CAD build for the part. Positions are in the model's coordinates, mm. A direction names the side the tool comes from. Round coordinates to 2 decimals unless told otherwise and drop trailing zeros. Write each loop counter-clockwise with the first axis right and the second up, starting at its lowest first coordinate (ties: lowest second). Pieces come first, ordered by that corner, then holes. Notation, with made-up numbers: (3, -9) - (27, -9) arc R17 cw to (27, 17) - close; hole circle Ø2 at (26.25, -8.75). An arc over 180 degrees is marked (long way). Answer in a Markdown table with one row per item.
```python
from build123d import *

# Parameters (mm, degrees)
ESQUISSE1_W                                        = 11
ESQUISSE1_H                                        = 26
BOSS_EXTRU_1_DEPTH                                 = 9
CHAMBRAGE_POUR_VIS_T_TE_RONDE_BOMB_E_M_D           = 3.4
CHAMBRAGE_POUR_VIS_T_TE_RONDE_BOMB_E_M_CBORE_D     = 7
CHAMBRAGE_POUR_VIS_T_TE_RONDE_BOMB_E_M_CBORE_DEPTH = 2.4
BOSS_EXTRU_2_DEPTH                                 = 40
DIAM_TRE_DU_PER_AGE_4_5_4_5_1_D                    = 4.5
ESQUISSE20_W                                       = 11
ESQUISSE20_H                                       = 28
ENL_V_MAT_EXTRU_6_DEPTH                            = 78.776924598
ESQUISSE21_W                                       = 50
ESQUISSE21_H                                       = 34
ENL_V_MAT_EXTRU_7_DEPTH                            = 72.960058366
ESQUISSE23_W                                       = 11
ESQUISSE23_H                                       = 14
BOSS_EXTRU_3_DEPTH                                 = 37
ESQUISSE24_W                                       = 37
ESQUISSE24_H                                       = 40
BOSS_EXTRU_4_DEPTH                                 = 3
ESQUISSE27_W                                       = 11
ESQUISSE27_H                                       = 37
ENL_V_MAT_EXTRU_11_DEPTH                           = 8
ESQUISSE28_W                                       = 64
ESQUISSE28_H                                       = 15
ENL_V_MAT_EXTRU_12_DEPTH                           = 6
ESQUISSE30_W                                       = 15
ESQUISSE30_H                                       = 8
ENL_V_MAT_EXTRU_13_DEPTH                           = 77.282370178
BOSS_EXTRU_6_DEPTH                                 = 3


with BuildPart() as part:
    # Esquisse1 → Boss.-Extru.1 (new body)
    with BuildSketch(Plane.XY):
        Rectangle(ESQUISSE1_W, ESQUISSE1_H)
    extrude(amount=BOSS_EXTRU_1_DEPTH)

    # Chambrage pour vis _ t_te ronde bomb_e M (through all)
    with Locations(Plane.XY.offset(9)):
        with Locations((0, 7.5), (0, -7.5)):
            CounterBoreHole(CHAMBRAGE_POUR_VIS_T_TE_RONDE_BOMB_E_M_D / 2, CHAMBRAGE_POUR_VIS_T_TE_RONDE_BOMB_E_M_CBORE_D / 2, CHAMBRAGE_POUR_VIS_T_TE_RONDE_BOMB_E_M_CBORE_DEPTH)

    # Esquisse8 → Boss.-Extru.2 (add)
    with BuildSketch(Plane.XZ.offset(13)):
        Polygon((-55.5, 0), (-55.5, 37), (5.5, 37), (5.5, 9), (-5.5, 9), (-5.5, 0), align=None)
    extrude(amount=-BOSS_EXTRU_2_DEPTH)

    # Diam_tre du per_age _4.5 _4.5_1 (through all)
    with Locations(Plane(origin=(0, 27, 0), x_dir=(1, 0, 0), z_dir=(0, 1, 0))):
        with Locations((-41.801370091, -19.00055804), (-18.801370091, -29.00055804)):
            Hole(DIAM_TRE_DU_PER_AGE_4_5_4_5_1_D / 2)

    # Esquisse20 → Enl_v. mat.-Extru.6 (cut, through all)
    with BuildSketch(Plane(origin=(0, 27, 0), x_dir=(1, 0, 0), z_dir=(0, 1, 0))):
        with Locations((0, -23)):
            Rectangle(ESQUISSE20_W, ESQUISSE20_H)
    extrude(amount=-ENL_V_MAT_EXTRU_6_DEPTH, mode=Mode.SUBTRACT)

    # Esquisse21 → Enl_v. mat.-Extru.7 (cut, through all)
    with BuildSketch(Plane.XY.offset(37)):
        with Locations((-30.5, 4)):
            Rectangle(ESQUISSE21_W, ESQUISSE21_H)
    extrude(amount=-ENL_V_MAT_EXTRU_7_DEPTH, mode=Mode.SUBTRACT)


with BuildPart() as enl_v_mat_extru_7_piece_1:
    # of the separate pieces the step leaves, piece 1, a body of its own (enl_v_mat_extru_7_pieces)
    add(part.part.solids().sort_by_distance((-5.5, 21, 0))[0])



with BuildPart() as enl_v_mat_extru_7_piece_2:
    # of the separate pieces the step leaves, piece 2, a body of its own (enl_v_mat_extru_7_pieces)
    add(part.part.solids().sort_by_distance((5.5, 13, 0))[0])


with BuildPart() as enl_v_mat_extru_7_piece_1_1:
    add(enl_v_mat_extru_7_piece_1.part)

    add(enl_v_mat_extru_7_piece_2.part)  # Boss.-Extru.3 merges Enl_v. mat.-Extru.7 piece 2
    # Esquisse23 → Boss.-Extru.3 (add, through all)
    with BuildSketch(Plane.XY.offset(37)):
        with Locations((0, 20)):
            Rectangle(ESQUISSE23_W, ESQUISSE23_H)
    extrude(amount=-BOSS_EXTRU_3_DEPTH)

    # Esquisse24 → Boss.-Extru.4 (add)
    with BuildSketch(Plane(origin=(5.5, 0, 0), x_dir=(0, 0, -1), z_dir=(1, 0, 0))):
        with Locations((-18.5, 7)):
            Rectangle(ESQUISSE24_W, ESQUISSE24_H)
    extrude(amount=BOSS_EXTRU_4_DEPTH)

    # Esquisse27 → Enl_v. mat.-Extru.11 (cut)
    with BuildSketch(Plane.XZ.offset(-21)):
        with Locations((0, 18.5)):
            Rectangle(ESQUISSE27_W, ESQUISSE27_H)
    extrude(amount=ENL_V_MAT_EXTRU_11_DEPTH, mode=Mode.SUBTRACT)

    # Esquisse28 → Enl_v. mat.-Extru.12 (cut)
    with BuildSketch(Plane(origin=(0, 27, 0), x_dir=(1, 0, 0), z_dir=(0, 1, 0))):
        with Locations((-23.5, -7.5)):
            Rectangle(ESQUISSE28_W, ESQUISSE28_H)
    extrude(amount=-ENL_V_MAT_EXTRU_12_DEPTH, mode=Mode.SUBTRACT)

    # Esquisse30 → Enl_v. mat.-Extru.13 (cut, through all)
    with BuildSketch(Plane.ZY.offset(-5.5)):
        with Locations((7.5, 17)):
            Rectangle(ESQUISSE30_W, ESQUISSE30_H)
    extrude(amount=-ENL_V_MAT_EXTRU_13_DEPTH, mode=Mode.SUBTRACT)

    # Esquisse31 → Boss.-Extru.6 (add, through all)
    with BuildSketch(Plane.ZY.offset(-5.5)):
        Polygon((15, 27), (0, 13), (15, 13), align=None)
    extrude(amount=-BOSS_EXTRU_6_DEPTH)


solid = enl_v_mat_extru_7_piece_1_1.part
```
Q1. Drill centre lines: line 1 (Y direction, x = 0, z = 7.25); line 2 (Y direction, x = 0, z = 2); line 3 (X direction, y = -10.5, z = 27.5). Where is each one in solid material? Low to high.
Computed:
| item | result |
|---|---|
| line 1 | y = -13 to -11, -4 to 4, 11 to 13 |
| line 2 | y = -13 to -9.2, -5.8 to 5.8, 9.2 to 13 |
| line 3 | x = 5.5 to 8.5 |
Q2. Saw through at D-D on y = 24. List the corners of the cut face in (x, z).
Computed:
| item | result |
|---|---|
| outline | (-55.5, 15) - (5.5, 15) - (5.5, 11.79) - (8.5, 11.79) - (8.5, 37) - (-55.5, 37) - close; hole circle Ø4.5 at (-41.8, 19); hole circle Ø4.5 at (-18.8, 29) |
Q3. 3-axis set-ups, long thin cutter, end or side, ignore diameter. For faces 1 (the flat face through (0, 13, 4)), 2 (the flat face through (-25, 21, 26)), 3 (the flat face through (2, 8, 6.6)): which of +Z, -Z, +X, -X, +Y, -Y reach the whole face in a straight line?
Computed:
| item | result |
|---|---|
| face 1 | +Z, -Z, -X, +Y |
| face 2 | +Z, -Z, -X, -Y |
| face 3 | +Z |
Q4. Saw through at B-B on y = -7.5. List the corners of the cut face in (x, z), then the cut area to 3 significant figures.
Computed:
| item | result |
|---|---|
| outline | (-5.5, 0) - (-1.7, 0) - (-1.7, 6.6) - (-3.5, 6.6) - (-3.5, 9) - (-5.5, 9) - close; (1.7, 0) - (8.5, 0) - (8.5, 37) - (5.5, 37) - (5.5, 9) - (3.5, 9) - (3.5, 6.6) - (1.7, 6.6) - close |
| area | 171 mm2 |
Q5. Saw through at C-C on z = 25.5. List the corners of the cut face in (x, y).
Computed:
| item | result |
|---|---|
| outline | (-55.5, 21) - (5.5, 21) - (5.5, -13) - (8.5, -13) - (8.5, 27) - (-55.5, 27) - close |
Q6. Flat gauge pins, fed straight in: pin 1 (2 mm diameter, centred on x = 1.5, y = -7.5, fed in from +Z); pin 2 (8 mm diameter, centred on y = 3, z = 28, fed in from -X); pin 3 (10 mm diameter, centred on x = -31.5, z = 26, fed in from -Y). Where does each tip first touch, or does it go through?
Computed:
| item | result |
|---|---|
| pin 1 | stops at z = 6.6 |
| pin 2 | stops at x = 5.5 |
| pin 3 | stops at y = 21 |
Q7. Saw through at A-A on x = 0. List the corners of the cut face in (y, z), then the cut area to 3 significant figures.
Computed:
| item | result |
|---|---|
| outline | (-13, 0) - (-9.2, 0) - (-9.2, 6.6) - (-11, 6.6) - (-11, 9) - (-13, 9) - close; (-5.8, 0) - (5.8, 0) - (5.8, 6.6) - (4, 6.6) - (4, 9) - (-4, 9) - (-4, 6.6) - (-5.8, 6.6) - close; (9.2, 0) - (13, 0) - (13, 9) - (11, 9) - (11, 6.6) - (9.2, 6.6) - close; (21, 15) - (27, 15) - (27, 37) - (21, 37) - close |
| area | 288 mm2 |
Q8. Pull direction Y, two halves, no side cores. Call faces 4 (the flat face through (8.5, 7, 18)), 5 (the flat face through (6.979, 20.098, 7.605)), 6 (the cylindrical face through (-0.759, -10.917, 7.817)): released by +Y, released by -Y, zero draft, split by the parting line, or undercut.
Computed:
| item | result |
|---|---|
| face 4 | zero draft |
| face 5 | released by +Y |
| face 6 | undercut |
